Part model, mm, in its own coordinate system. A direction names the side the tool comes from. Give positions to 0.01 mm unless a question says otherwise; leave off trailing zeros. Order: outer loops, then holes, each group sorted by start corner. A loop starts at its lowest first (then second) coordinate and runs counter-clockwise, first axis right, second up. Notation, with made-up numbers: (76.5, 48) - (89.5, 48) arc R16 cw to (89.5, 78) - close; hole circle Ø3 at (82.25, -34.5). An arc over 180 degrees is marked (long way). One line per item, written item: value.
```python
from build123d import *

# Parameters (mm, degrees)
SKETCH1_R           = 1.5
BOSS_EXTRUDE1_DEPTH = 3


with BuildPart() as part:
    # Sketch1 → Boss-Extrude1 (new body)
    with BuildSketch(Plane.XY):
        with BuildLine():
            Line((28.6, 0), (28.6, 18.3))
            ThreePointArc((28.6, 18.3), (27.721320344, 20.421320344), (25.6, 21.3))
            Line((25.6, 21.3), (0, 21.3))
            ThreePointArc((0, 21.3), (-2.121320344, 20.421320344), (-3, 18.3))
            Line((-3, 18.3), (-3, 0))
            ThreePointArc((-3, 0), (-2.121320344, -2.121320344), (0, -3))
            Line((0, -3), (25.6, -3))
            ThreePointArc((25.6, -3), (27.721320344, -2.121320344), (28.6, 0))
        make_face()
        with Locations((11.8, 0.15)):
            Circle(SKETCH1_R, mode=Mode.SUBTRACT)
        with Locations((13.3, 19.35)):
            Circle(SKETCH1_R, mode=Mode.SUBTRACT)
        Polygon((24.7, 3.2), (24.7, 16), (1.6, 16), (1.6, 12.1), (-0.4, 12.1), (-0.4, 7.1), (1.6, 7.1), (1.6, 3.2), align=None, mode=Mode.SUBTRACT)
    extrude(amount=BOSS_EXTRUDE1_DEPTH)


solid = part.part
```
1) Mould opens along X. For faces 1 (the flat face through (13, 17, 3)), 2 (the flat face through (24.7, 10, 1)), 3 (the cylindrical face through (-2.1, 20.44, 1.48)) say: released by +X, released by -X, zero draft, split by the parting line, or undercut.
Outcome:
face 1: zero draft
face 2: undercut
face 3: released by -X
2) Pin check, flat tip, straight feed: pin 1 (3 mm diameter, centred on x = 3.5, y = 11, fed in from -Z). Stop position of the tip, or through.
Outcome:
pin 1: passes through
3) Cut at B-B, the plane x = 4. Give the cut face in (y, z), then the cut area to 3 significant figures.
Outcome:
outline: (-3, 0) - (3.2, 0) - (3.2, 3) - (-3, 3) - close; (16, 0) - (21.3, 0) - (21.3, 3) - (16, 3) - close
area: 34.5 mm^2
4) Drill centre lines: line 1 along Y through (x, z) = (18.5, 1.6); line 2 along Y through (x, z) = (13.5, 1.15); line 3 along X through (y, z) = (12.5, 2.35). Where is each one in solid material? Low to high. Write a range as from..to.
Outcome:
line 1: y = -3..3.2, 16..21.3
line 2: y = -3..3.2, 16..17.86, 20.84..21.3
line 3: x = -3..1.6, 24.7..28.6
5) Cut at A-A, the plane y = 19.35. Give the cut face in (x, z).
Outcome:
outline: (-2.81, 0) - (11.8, 0) - (11.8, 3) - (-2.81, 3) - close; (14.8, 0) - (28.41, 0) - (28.41, 3) - (14.8, 3) - close
6) Cut at C-C, the plane z = 1.25. Give the cut face in (x, y), then the cut area to 3 significant figures.
Outcome:
outline: (-3, 0) arc R3 ccw to (0, -3) - (25.6, -3) arc R3 ccw to (28.6, 0) - (28.6, 18.3) arc R3 ccw to (25.6, 21.3) - (0, 21.3) arc R3 ccw to (-3, 18.3) - close; hole (-0.4, 7.1) - (1.6, 7.1) - (1.6, 3.2) - (24.7, 3.2) - (24.7, 16) - (1.6, 16) - (1.6, 12.1) - (-0.4, 12.1) - close; hole circle Ø3 at (11.8, 0.15); hole circle Ø3 at (13.3, 19.35)
area: 440 mm^2
7) Which spindle directions (+Z, -Z, +X, -X, +Y, -Y) get a long thin tool onto all of the face, cutting with end or side? Do faces 4 (the flat face through (13, 3.2, 1)), 5 (the cylindrical face through (-2.14, -2.1, 1.48)). Say none if no direction does.
Outcome:
face 4: +Z, -Z
face 5: +Z, -Z, -X, -Y
